from build123d import *

# Parameters (mm, degrees)
F1_DEPTH = 101.6
F2_R     = 6.34999
F3_R     = 3.175
F4_DEPTH = 25.4
F6_DEPTH = 25.4


# Not quite as in the source:
# - a fillet or chamfer is up to 0.001 mm smaller than in the source, because OpenCascade refuses the exact size


with BuildPart() as f1:
    # F0 (on Front) → F1 (new body)
    with BuildSketch(Plane.XZ):
        Polygon((-79.5245949868, 52.4404040542), (-85.8745949868, 52.4404040542), (-85.8745949868, -61.8595959458), (28.4254050132, -61.8595959458), (28.4254050132, -55.5095959458), (-79.5245949868, -55.5095959458), align=None)
    extrude(amount=F1_DEPTH)

    # F2 (radius 6.35 in the source; OpenCascade refuses exactly that, so slightly less here)
    f2_edges = [f1.edges().sort_by_distance(p)[0] for p in [
        (-79.524595, -50.8, 52.440404),
        (28.425405, -50.8, -55.509596),
        (-79.524595, -50.8, -55.509596),
    ]]
    fillet(f2_edges, radius=F2_R)

    # F3 (on face) → F4 (cut)
    with BuildSketch(Plane.YZ.offset(-79.5245949868)):
        with BuildLine():
            Line((-39.7764292627, 21.6810040542), (-61.8235707373, 21.6810040542))
            ThreePointArc((-61.8235707373, 21.6810040542), (-50.8, -33.3099959458), (-39.7764292627, 21.6810040542))
        make_face()
        with Locations((-87.5792, -4.7095959458)):
            Circle(F3_R)
        with Locations((-14.0208, -4.7095959458)):
            Circle(F3_R)
    extrude(amount=-F4_DEPTH, mode=Mode.SUBTRACT)

    # F5 (on face) → F6 (cut)
    with BuildSketch(Plane.XY.offset(-55.5095959458)):
        with BuildLine():
            ThreePointArc((-57.1725949868, -72.263), (-61.1095949868, -76.2), (-57.1725949868, -80.137))
            Line((-57.1725949868, -80.137), (11.1534050132, -80.137))
            ThreePointArc((11.1534050132, -80.137), (15.0904050132, -76.2), (11.1534050132, -72.263))
            Line((11.1534050132, -72.263), (-57.1725949868, -72.263))
        make_face()
        with BuildLine():
            ThreePointArc((-57.1725949868, -21.463), (-61.1095949868, -25.4), (-57.1725949868, -29.337))
            Line((-57.1725949868, -29.337), (11.1534050132, -29.337))
            ThreePointArc((11.1534050132, -29.337), (15.0904050132, -25.4), (11.1534050132, -21.463))
            Line((11.1534050132, -21.463), (-57.1725949868, -21.463))
        make_face()
    extrude(amount=-F6_DEPTH, mode=Mode.SUBTRACT)


solid = f1.part
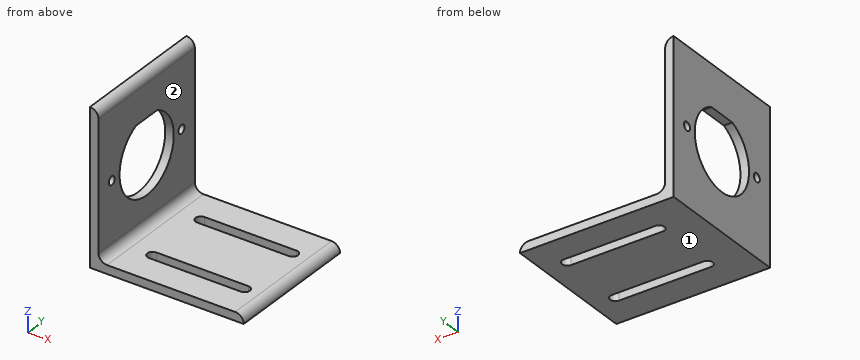
Check sheet for the modelled part. Datum: model origin and axes. Units: mm. Face numbers are marked on the shaded views. A direction names the side the tool comes from. Round coordinates to 2 decimals unless told otherwise and drop trailing zeros. Order: outer loops, then holes, each group sorted by start corner. A loop starts at its lowest first (then second) coordinate and runs counter-clockwise, first axis right, second up.
Q1. Depth check by flat-ended pin: P1, Ø10, axis at y = -87.58, z = -4.71, coming from the +X side; P2, Ø8, axis at x = -19, y = -60, coming from the +Z side; P3, Ø6, axis at y = -45.5, z = -28.5, coming from the +X side; P4, Ø1.5, axis at x = -33.5, y = -21.5, coming from the -Z side. Enter the tip coordinate at first touch or a pass-through.
Filled sheet:
P1: stops at x = -79.52
P2: stops at z = -55.51
P3: passes through
P4: stops at z = -61.86
Q2. Set-up check for the marked faces 1 and 2: record each of +Z, -Z, +X, -X, +Y, -Y from which the full face is reachable in a straight line by a thin tool's end or side.
Filled sheet:
face 1: -Z, +X, -X, +Y, -Y
face 2: +Z, +X, +Y, -Y
Q3. Scan lines: L1, parallel to Z at x = 3.5, y = -57; L2, parallel to X at y = -18, z = -16; L3, parallel to Z at x = -82.5, y = -50.8. Record each from-to range of solid material in increasing order.
Filled sheet:
L1: z = -61.86 to -55.51
L2: x = -85.87 to -79.52
L3: z = -61.86 to -33.31, 21.68 to 51.47
Q4. Cross-section at B-B, the plane x = -32. Enter the section's corners in (y, z).
Filled sheet:
outline: (-101.6, -61.86) - (-80.14, -61.86) - (-80.14, -55.51) - (-101.6, -55.51) - close; (-72.26, -61.86) - (-29.34, -61.86) - (-29.34, -55.51) - (-72.26, -55.51) - close; (-21.46, -61.86) - (0, -61.86) - (0, -55.51) - (-21.46, -55.51) - close
Q5. Cross-section at D-D, the plane z = -30.5. Enter the section's corners in (x, y), plus the area to 3 significant figures.
Filled sheet:
outline: (-85.87, -101.6) - (-79.52, -101.6) - (-79.52, -63.16) - (-85.87, -63.16) - close; (-85.87, -38.44) - (-79.52, -38.44) - (-79.52, 0) - (-85.87, 0) - close
area: 488 mm2
